Autodesk Inventor part; units mm, degrees
ref_plane "YZ Plane" through (0, 0, 0) normal (1, 0, 0) x (0, 1, 0)
ref_plane "XZ Plane" through (0, 0, 0) normal (0, 1, 0) x (-1, 0, 0)
ref_plane "XY Plane" through (0, 0, 0) normal (0, 0, 1) x (1, 0, 0)
sketch "Esquisse1" plane through (0, 0, 0) normal (0, 1, 0) x (-1, 0, 0)
  line L0 (-1.5, 50) -> (1.5, 50)
  line L1 (1.5, 50) -> (1.5, -50)
  line L2 (1.5, -50) -> (-1.5, -50)
  line L3 (-1.5, -50) -> (-1.5, 50)
  line L4 (1.5, 50) -> (-1.5, -50)
  line L5 (-1.5, 50) -> (1.5, -50)
  circle A0 centre (14, -35) radius 12.5
  line L6 (-10, 0) -> (16, 0)
  circle A1 centre (14, 35) radius 12.5
  line L7 (1.5, -50) -> (14, -50)
  line L8 (14, -50) -> (14, -47.5)
  line L9 (9, -23.5436) -> (9, 23.5436)
  line L10 (1.5, 50) -> (14.5259, 50)
  line L11 (14.5259, 50) -> (14.5259, 47.4889)
  point P0 (0, 0)
  point P1 (0, 0)
  point P2 (0, 0)
  point P3 (14, -22.5)
  point P4 (14, 22.5)
  point P5 (1.5, 35)
  point P6 (1.5, -35)
  dimension "d0" = 3
  dimension "d1" = 100
  dimension "d19" = 25
extrude "Extrusion1" add sketch "Esquisse1" along normal blind 10 contours L5 L6 L3 | L0 L4 L5 | L10 L11 A1 L1 | L1 L6 L4 | L6 L4 L3 | L5 L2 L4 | L6 L1 L5 | L1 A0 L8 L7
sketch "Esquisse2" plane through (1.5, 0, 50) normal (1, 0, 0) x (0, 0, -1)
  line L0 (0, 0) -> (100, 0)
  line L1 (27.9472, 0) -> (32.9472, 0)
  line L2 (32.9472, 0) -> (32.9472, 10)
  line L3 (32.9472, 10) -> (27.9472, 10)
  line L4 (27.9472, 10) -> (27.9472, 0)
  line L5 (50, 0) -> (50, 10.1076)
  line L6 (67.0528, 0) -> (67.0528, 10)
  line L7 (67.0528, 10) -> (72.0528, 10)
  line L8 (72.0528, 10) -> (72.0528, 0)
  dimension "d4" = 5
  dimension "d5" = 10
extrude "Extrusion2" add sketch "Esquisse2" along normal blind 15
fillet "Congé1" radius 10 2 edges at (1.5, 5, -50) (1.5, 5, 50)
sketch "Esquisse5" plane through (0, 10, 0) normal (0, 1, 0) x (1, 0, 0)
  line L0 (16.5, 17.0528) -> (16.5, 22.0528)
  line L1 (1.5, 17.0528) -> (16.5, 17.0528)
  line L2 (16.5, 22.0528) -> (11.5, 22.0528)
  line L3 (11.5, 22.0528) -> (11.5, 17.0528)
  line L4 (11.5, 17.0528) -> (16.5, 17.0528)
  line L5 (16.5, 17.0528) -> (16.5, 22.0528)
  line L6 (-9, 0) -> (10, 0)
  line L7 (16.5, -17.0528) -> (16.5, -22.0528)
  line L8 (16.5, -22.0528) -> (11.5, -22.0528)
  line L9 (11.5, -22.0528) -> (11.5, -17.0528)
  line L10 (11.5, -17.0528) -> (16.5, -17.0528)
  line L11 (16.5, -17.0528) -> (16.5, -22.0528)
  point P0 (0, 0)
  dimension "d22" = 5
extrude "Extrusion5" add sketch "Esquisse5" along normal blind 10
sketch "Esquisse6" plane through (16.5, 0, 50) normal (1, 0, 0) x (0, 0, -1)
  circle A0 centre (30.4472, 15) radius 1.75
  line L0 (27.9472, 20) -> (32.9472, 20)
  line L1 (27.9472, 0) -> (27.9472, 20)
  line L2 (50, 0) -> (50, 10)
  circle A1 centre (69.5528, 15) radius 1.75
  point P0 (30.4472, 20)
  dimension "d25" = 3.5
  dimension "d26" = 5
  dimension "d27" = 2.5
extrude "Extrusion6" cut sketch "Esquisse6" against normal blind 10
fillet "Congé2" radius 5 6 edges at (16.5, 0, 19.5528) (16.5, 0, -19.5528) (1.5, 5, 22.0528) (1.5, 5, -22.0528) (1.5, 5, -17.0528) (1.5, 5, 17.0528)
fillet "Congé3" radius 2 2 edges at (11.5, 20, 19.5528) (11.5, 20, -19.5528)
sketch "Esquisse7" plane through (0, 10, 0) normal (0, 1, 0) x (1, 0, 0)
  circle A0 centre (2, 19.5528) radius 1.75
  line L0 (-3.6278, 0) -> (5, 0)
  circle A1 centre (2, -19.5528) radius 1.75
  line L1 (6.5, 22.0528) -> (11.5, 22.0528)
  point P0 (0, 0)
  dimension "d32" = 3.5
  dimension "d33" = 2.5
extrude "Extrusion7" cut sketch "Esquisse7" against normal blind 23
sketch "Esquisse8" plane through (1.5, 0, 12.0528) normal (1, 0, 0) x (0, 0, -1)
  circle A0 centre (7.0528, 5) radius 1.75
  line L0 (12.0528, 0) -> (12.0528, 10)
  circle A1 centre (17.0528, 5) radius 1.75
  point P0 (12.0528, 5)
  dimension "d36" = 3.5
  dimension "d37" = 5
extrude "Extrusion8" cut sketch "Esquisse8" against normal blind 3
properties part number "pare-chocs"
Read the model definition and answer for the solid it produces. Units are mm, in the model's axes. A direction names the side the tool comes from. Coordinates: 2 decimals unless noted, no trailing zeros. Write each loop counter-clockwise with the first axis right and the second up, starting at its lowest first coordinate (ties: lowest second). Pieces come first, ordered by that corner, then holes. Notation, with made-up numbers: M -11.5,29.5 L -5.5,29.5 A17 ccw -5.5,51.5 Z; hole C 51.5,-3 d11. An arc over 180 degrees is marked long. Use a Markdown table: item, result.
Q1. Determine the mould class of faces 1 (the face through (-14.526, 5, 49)), 2 (the face through (13, 8, -17.053)), 3 (the face through (14.035, 16.735, -19.325)), 4 (the face through (13, 8, 22.053)) for opening direction Z: released by +Z, released by -Z, zero draft, split by the parting line, or undercut.
Answer block:
| item | result |
|---|---|
| face 1 | zero draft |
| face 2 | undercut |
| face 3 | undercut |
| face 4 | released by +Z |
Q2. Each of these flat-tipped pins is pushed along its axis until it touches: pin 1 Ø10 at (y, z) = (9, 20) entering from -X; pin 2 Ø3 at (x, y) = (12, 13.5) entering from +Z; pin 3 Ø5 at (x, y) = (5.5, 10.5) entering from -Z; pin 4 Ø2 at (y, z) = (5, -5) entering from +X. Where does it stop, or does it pass through?
Answer block:
| item | result |
|---|---|
| pin 1 | stops at x = -1.5 |
| pin 2 | stops at z = 22.05 |
| pin 3 | stops at z = -23.43 |
| pin 4 | passes through |
Q3. Straight lines are drawn through the part: L1, parallel to Z at x = 14, y = 1.5; L2, parallel to Z at x = 2, y = 5.75; L3, parallel to Y at x = 0, z = 5. For each, find the intervals that lie inside material, in ascending order. Write a range as [from, to].
Answer block:
| item | result |
|---|---|
| L1 | z = [-22.05, -17.05], [17.05, 22.05] |
| L2 | z = [-24.87, -21.3], [-17.8, -14.23], [14.23, 17.8], [21.3, 24.87] |
| L3 | y = [0, 3.25], [6.75, 10] |
Q4. The part is cut by section C-C, the plane z = 5. Write down the section's boundary in (x, y), then the cut area to 3 significant figures.
Answer block:
| item | result |
|---|---|
| outline | M -1.5,0 L 1.5,0 L 1.5,3.25 L -1.5,3.25 Z; M -1.5,6.75 L 1.5,6.75 L 1.5,10 L -1.5,10 Z |
| area | 19.5 mm2 |
Q5. The part is cut by section D-D, the plane x = -11. Write down the section's boundary in (y, z).
Answer block:
| item | result |
|---|---|
| outline | M 0,-50 L 10,-50 L 10,-47.13 L 0,-47.13 Z; M 0,47.13 L 10,47.13 L 10,50 L 0,50 Z |
Q6. Which of the six approach directions +Z, -Z, +X, -X, +Y, -Y give full straight-line access (tool end or side, diameter ignored) to faces 5 (the face through (1.5, 5, -34)), 6 (the face through (-5.259, 4.93, -43.935)), 7 (the face through (-14, 5, -49)), 8 (the face through (3.004, 5.07, -15.627))?
Answer block:
| item | result |
|---|---|
| face 5 | -Z, +X, +Y, -Y |
| face 6 | -X, +Y, -Y |
| face 7 | -Z, -X, +Y, -Y |
| face 8 | +X, +Y, -Y |
Q7. The part is cut by section A-A, the plane y = 15. Write down the section's boundary in (x, z), then the cut area to 3 significant figures.
Answer block:
| item | result |
|---|---|
| outline | M 11.5,-22.05 L 16.5,-22.05 L 16.5,-21.3 L 11.5,-21.3 Z; M 11.5,-17.8 L 16.5,-17.8 L 16.5,-17.05 L 11.5,-17.05 Z; M 11.5,17.05 L 16.5,17.05 L 16.5,17.8 L 11.5,17.8 Z; M 11.5,21.3 L 16.5,21.3 L 16.5,22.05 L 11.5,22.05 Z |
| area | 15.0 mm2 |
Q8. The part is cut by section B-B, the plane x = 2.5. Write down the section's boundary in (y, z), then the cut area to 3 significant figures.
Answer block:
| item | result |
|---|---|
| outline | M 0,-24.05 L 10,-24.05 L 10,-21.23 L 0,-21.23 Z; M 0,-17.88 L 10,-17.88 L 10,-15.05 L 0,-15.05 Z; M 0,15.05 L 10,15.05 L 10,17.88 L 0,17.88 Z; M 0,21.23 L 10,21.23 L 10,24.05 L 0,24.05 Z |
| area | 113 mm2 |
